Here's how the part is built. I have some questions about the finished solid (model axes, mm). A direction names the side the tool comes from. Coordinates: 2 decimals unless noted, no trailing zeros. Order: outer loops, then holes, each group sorted by start corner. A loop starts at its lowest first (then second) coordinate and runs counter-clockwise, first axis right, second up. Notation, with made-up numbers: (18.5, 87.5) - (34.5, 87.5) arc R21 cw to (34.5, 115.5) - close; hole circle Ø8 at (14, 72.25). An arc over 180 degrees is marked (long way). Answer as CSV lines item,"result". Start each with the question number.
Item 1: We'd pull the mould along X, two halves only. Please class faces 1 (the face through (-35, -18.52, 0)), 2 (the face through (-6.67, 5.97, -0.11)), 3 (the face through (6.819, 5.815, -0.105)), 4 (the face through (-3, -12, -7.5)): pulls with the +X half, pulls with the -X half, needs draft (parallel to the pull), parting line crosses it, or undercut.
Item 2: Imagine slicing it at C-C on y = 0. List the corners of the cut face in (x, z) for me, and give its area (3 significant figures).
Item 3: Imagine slicing it at A-A on z = -3.5. List the corners of the cut face in (x, y) for me, and give its area (3 significant figures).
Item 4: I'm going to push flat-ended pins straight in: pin 1 (17 mm diameter, centred on x = 0, y = 0, fed in from -Z); pin 2 (1.5 mm diameter, centred on x = -32.5, y = -8.5, fed in from -Z); pin 3 (1.5 mm diameter, centred on x = -24.5, z = -6, fed in from +Y). Where does each tip first touch, or does it pass through?
Item 5: On a 3-axis mill with a long thin cutter (end or side, diameter ignored), from which of +Z, -Z, +X, -X, +Y, -Y can I reach the whole of each face in a straight line? I mean faces 5 (the face through (3, 0, 2.5)), 6 (the face through (-3, -12, 7.5)), 7 (the face through (-25, -13.52, 0)), 8 (the face through (3, 0, -2.5)). Say none if no direction works.
Item 6: Imagine slicing it at D-D on y = 3.5. List the corners of the cut face in (x, z) for me, and give its area (3 significant figures).
Item 7: I need wall thicknesses on line 1 (Y direction, x = 0, z = -3.7); line 2 (Z direction, x = -30, y = -9); line 3 (X direction, y = -14.5, z = -0.25). Which ranges of each line are inside material? Lowest first, please.
Item 8: Imagine slicing it at B-B on x = -33. List the corners of the cut face in (y, z) for me, and give its area (3 significant figures).
from build123d import *

# Parameters (mm, degrees)
SKETCH1_R               = 6.52
SKETCH1_R_2             = 2.25
BOSS_EXTRUDE1_DEPTH     = 7.5
CUT_EXTRUDE1_START      = 7.5
SKETCH1_3_R             = 6.52
CUT_EXTRUDE1_DEPTH      = 5
CUT_EXTRUDE2_START      = -2.5
SKETCH1_4_R             = 6.52
CUT_EXTRUDE2_DEPTH      = 5
SKETCH2_R               = 14.4
BOSS_EXTRUDE2_DEPTH     = 19
CUT_EXTRUDE3_DEPTH      = 51.395634732
CUT_EXTRUDE3_DEPTH_BACK = 51.395634732
CUT_EXTRUDE4_DEPTH      = 7
CUT_EXTRUDE5_START      = -12
SKETCH2_5_R             = 11.4
CUT_EXTRUDE5_DEPTH      = 7
FILLET1_R               = 5
FILLET2_R               = 10


with BuildPart() as part:
    # Sketch1 → Boss-Extrude1 (new, symmetric)
    # profile 1 of 3: a face of its own
    with BuildSketch(Plane.XY):
        Polygon((-4.7e-08, -6.52), (-9.5, -6.52), (-16.20264212, -6.52), (-30, -6.52), (-30, -25.52), (9.5, -25.52), (9.5, -6.52), align=None)
    # profile 2 of 3: a face of its own
    with BuildSketch(Plane.XY):
        Polygon((9.5, 9), (-9.5, 9), (-9.5, -6.52), (-4.7e-08, -6.52), (9.5, -6.52), align=None)
        with BuildLine():
            ThreePointArc((6.52, 0), (4.610336197, -4.61033623), (-4.7e-08, -6.52))
            ThreePointArc((-4.7e-08, -6.52), (-4.610336197, 4.61033623), (6.52, 0))
        make_face(mode=Mode.SUBTRACT)
    # profile 3 of 3: a face of its own
    with BuildSketch(Plane.XY):
        Circle(SKETCH1_R)
        Circle(SKETCH1_R_2, mode=Mode.SUBTRACT)
    extrude(amount=BOSS_EXTRUDE1_DEPTH, both=True)

    # Sketch1<3> → Cut-Extrude1 (cut)
    with BuildSketch(Plane.XY.offset(CUT_EXTRUDE1_START)):
        Circle(SKETCH1_3_R)
    extrude(amount=-CUT_EXTRUDE1_DEPTH, mode=Mode.SUBTRACT)

    # Sketch1<4> → Cut-Extrude2 (cut)
    with BuildSketch(Plane.XY.offset(CUT_EXTRUDE2_START)):
        Circle(SKETCH1_4_R)
    extrude(amount=-CUT_EXTRUDE2_DEPTH, mode=Mode.SUBTRACT)

    # Sketch2 → Boss-Extrude2 (add, through all)
    with BuildSketch(Plane(origin=(0, -6.52, 0), x_dir=(1, 0, 0), z_dir=(0, 1, 0))):
        with Locations((-30, 0)):
            Circle(SKETCH2_R)
    extrude(amount=-BOSS_EXTRUDE2_DEPTH)

    # Sketch2<3> → Cut-Extrude3 (cut, two sides: drawn at the far end of the back side and taken through both)
    with BuildSketch(Plane(origin=(0, -6.52, 0), x_dir=(1, 0, 0), z_dir=(0, 1, 0)).offset(-CUT_EXTRUDE3_DEPTH_BACK)):
        with BuildLine():
            ThreePointArc((-30, -4.25), (-26.99479618, -3.00520382), (-25.75, 0))
            ThreePointArc((-25.75, 0), (-26.99479618, 3.00520382), (-30, 4.25))
            Line((-30, 4.25), (-30, -4.25))
        make_face()
        with BuildLine():
            Line((-30, -4.25), (-30, 4.25))
            ThreePointArc((-30, 4.25), (-34.25, 0), (-30, -4.25))
        make_face()
    extrude(amount=CUT_EXTRUDE3_DEPTH + CUT_EXTRUDE3_DEPTH_BACK, mode=Mode.SUBTRACT)

    # Sketch2<4> → Cut-Extrude4 (cut)
    with BuildSketch(Plane(origin=(0, -6.52, 0), x_dir=(1, 0, 0), z_dir=(0, 1, 0))):
        with BuildLine():
            ThreePointArc((-21.414547187, -7.5), (-19.326805491, -4.005361278), (-18.6, 0))
            ThreePointArc((-18.6, 0), (-19.326805491, 4.005361278), (-21.414547187, 7.5))
            Line((-21.414547187, 7.5), (-30, 7.5))
            Line((-30, 7.5), (-30, 4.25))
            ThreePointArc((-30, 4.25), (-26.99479618, 3.00520382), (-25.75, 0))
            ThreePointArc((-25.75, 0), (-26.99479618, -3.00520382), (-30, -4.25))
            Line((-30, -4.25), (-30, -7.5))
            Line((-30, -7.5), (-21.414547187, -7.5))
        make_face()
        with BuildLine():
            Line((-30, 7.5), (-21.414547187, 7.5))
            ThreePointArc((-21.414547187, 7.5), (-41.4, 0), (-21.414547187, -7.5))
            Line((-21.414547187, -7.5), (-30, -7.5))
            Line((-30, -7.5), (-30, -4.25))
            ThreePointArc((-30, -4.25), (-34.25, 0), (-30, 4.25))
            Line((-30, 4.25), (-30, 7.5))
        make_face()
    extrude(amount=-CUT_EXTRUDE4_DEPTH, mode=Mode.SUBTRACT)

    # Sketch2<5> → Cut-Extrude5 (cut)
    with BuildSketch(Plane(origin=(0, -6.52, 0), x_dir=(1, 0, 0), z_dir=(0, 1, 0)).offset(CUT_EXTRUDE5_START)):
        with Locations(Location((-30, 0, 0), (0, 0, 270))):
            Circle(SKETCH2_5_R)
    extrude(amount=-CUT_EXTRUDE5_DEPTH, mode=Mode.SUBTRACT)

    # Fillet1
    fillet1_edges = [part.edges().sort_by_distance(p)[0] for p in [
        (-9.5, -6.52, 0),
        (-17.707319251, -16.02, -7.5),
        (-17.707319251, -16.02, 7.5),
    ]]
    fillet(fillet1_edges, radius=FILLET1_R)

    # Fillet2
    # the kernel refuses this fillet: 10 mm, written as the material it takes off along each edge
    with BuildSketch(Plane(origin=(-9.5, 9, -32.5), x_dir=(0, -1, 0), z_dir=(0, 0, 1)), Plane(origin=(9.5, 9, -32.5), x_dir=(-1, 0, 0), z_dir=(0, 0, 1)), Plane(origin=(9.5, -25.52, 32.5), x_dir=(-1, 0, 0), z_dir=(0, 0, -1))) as fillet2_piece_1:
        with BuildLine():
            CenterArc((FILLET2_R, FILLET2_R), FILLET2_R, 180, 90)
            Line((0, FILLET2_R), (0, 0))
            Line((0, 0), (FILLET2_R, 0))
        make_face()
    extrude(amount=65, mode=Mode.SUBTRACT)


solid = part.part
Responses:
1,face 1,"undercut"
1,face 2,"pulls with the -X half"
1,face 3,"pulls with the +X half"
1,face 4,"needs draft"
2,outline,"(-9.45, -7.5) - (-6.52, -7.5) - (-6.52, -2.5) - (-2.25, -2.5) - (-2.25, 2.5) - (-6.52, 2.5) - (-6.52, 7.5) - (-9.45, 7.5) - close; (2.25, -2.5) - (6.52, -2.5) - (6.52, -7.5) - (9.45, -7.5) - (9.45, 7.5) - (6.52, 7.5) - (6.52, 2.5) - (2.25, 2.5) - close"
2,area,"131 mm^2"
3,outline,"(-43.97, -25.52) - (-40.85, -25.52) - (-40.85, -18.52) - (-32.41, -18.52) - (-32.41, -13.52) - (-40.85, -13.52) - (-40.85, -6.52) - (-43.97, -6.52) - close; (-27.59, -18.52) - (-19.15, -18.52) - (-19.15, -25.52) - (-0.5, -25.52) arc R10 ccw to (9.5, -15.52) - (9.5, -1) arc R10 ccw to (0, 8.99) arc R10 ccw to (-9.5, -1) - (-9.5, -1.52) arc R5 cw to (-14.5, -6.52) - (-19.15, -6.52) - (-19.15, -13.52) - (-27.59, -13.52) - close; hole circle Ø13.04 at (0, 0)"
3,area,"790 mm^2"
4,pin 1,"stops at z = -7.5"
4,pin 2,"stops at z = -14.29"
4,pin 3,"stops at y = -13.52"
5,face 5,"+Z"
5,face 6,"+Z, +X, +Y, -Y"
5,face 7,"+Y"
5,face 8,"-Z"
6,outline,"(-8.43, -7.5) - (-5.5, -7.5) - (-5.5, -2.5) - (5.5, -2.5) - (5.5, -7.5) - (8.43, -7.5) - (8.43, 7.5) - (5.5, 7.5) - (5.5, 2.5) - (-5.5, 2.5) - (-5.5, 7.5) - (-8.43, 7.5) - close"
6,area,"143 mm^2"
7,line 1,"y = -25.51 to -6.52, 6.52 to 8.99"
7,line 2,"z = -14.4 to -11.4, 11.4 to 14.4"
7,line 3,"x = -44.4 to -34.24, -25.76 to 9.5"
8,outline,"(-25.52, -14.08) - (-6.52, -14.08) - (-6.52, -11) - (-13.52, -11) - (-13.52, -3.01) - (-18.52, -3.01) - (-18.52, -11) - (-25.52, -11) - close; (-25.52, 11) - (-18.52, 11) - (-18.52, 3.01) - (-13.52, 3.01) - (-13.52, 11) - (-6.52, 11) - (-6.52, 14.08) - (-25.52, 14.08) - close"
8,area,"197 mm^2"
